```python
from build123d import *

# Parameters (mm, degrees)
SKETCH2_R           = 10
BOSS_EXTRUDE1_DEPTH = 50


with BuildPart() as part:
    # Sketch2 → Boss-Extrude1 (new body)
    with BuildSketch(Plane.XY):
        with BuildLine():
            Line((0, 40), (1000, 40))
            ThreePointArc((1000, 40), (1040, 0), (1000, -40))
            Line((1000, -40), (0, -40))
            ThreePointArc((0, -40), (-40, 0), (0, 40))
        make_face()
        Circle(SKETCH2_R, mode=Mode.SUBTRACT)
    extrude(amount=-BOSS_EXTRUDE1_DEPTH)


solid = part.part
```
The listing builds one solid part. Answer for the finished solid, in the listing's coordinates (mm). Round coordinates to 2 decimals unless told otherwise and drop trailing zeros. Loops run counter-clockwise (first coordinate to the right, second up) from the corner with the lowest first, then second, coordinate; pieces in that order, holes last.
Q1. Section B-B, the plane z = -25.5 is taken. Determine the outline of the cut face in (x, y), then the cut area to 3 significant figures.
Q2. Given pin 1 Ø1.5 at (y, z) = (28, -41.5) entering from -X; pin 2 Ø18 at (x, y) = (0, 0) entering from +Z; pin 3 Ø8 at (y, z) = (15, -26) entering from -X; pin 4 Ø8 at (y, z) = (7.5, -42) entering from -X, each flat-ended and moving along its own axis, determine where each tip first touches the part or whether it passes through.
Q3. Find the intervals of material crossed by line 1 (Y direction, x = 0, z = -14.5); line 2 (X direction, y = 3, z = -37); line 3 (X direction, y = 34.5, z = -33), in increasing order.
Q4. Section A-A, the plane y = 0 is taken. Determine the outline of the cut face in (x, z), then the cut area to 3 significant figures.
Q5. For a pull along Y with two mould halves and no side action, classify faces 1 (the face through (508, 1, -50)), 2 (the face through (507, -40, -25)), 3 (the face through (-2.17, -9.76, -24.65)) as released by +Y, released by -Y, zero draft, split by the parting line, or undercut.
Completed:
1. outline: (0, -40) - (1000, -40) arc R40 ccw to (1000, 40) - (0, 40) arc R40 ccw to start; hole circle Ø20 at (0, 0)
1. area: 84,700 mm2
2. pin 1: stops at x = -29.28
2. pin 2: passes through
2. pin 3: stops at x = -38.46
2. pin 4: stops at x = -39.85
3. line 1: y = -40 to -10, 10 to 40
3. line 2: x = -39.89 to -9.54, 9.54 to 1039.89
3. line 3: x = -20.24 to 1020.24
4. outline: (-40, -50) - (-10, -50) - (-10, 0) - (-40, 0) - close; (10, -50) - (1040, -50) - (1040, 0) - (10, 0) - close
4. area: 53,000 mm2
5. face 1: zero draft
5. face 2: released by -Y
5. face 3: undercut
